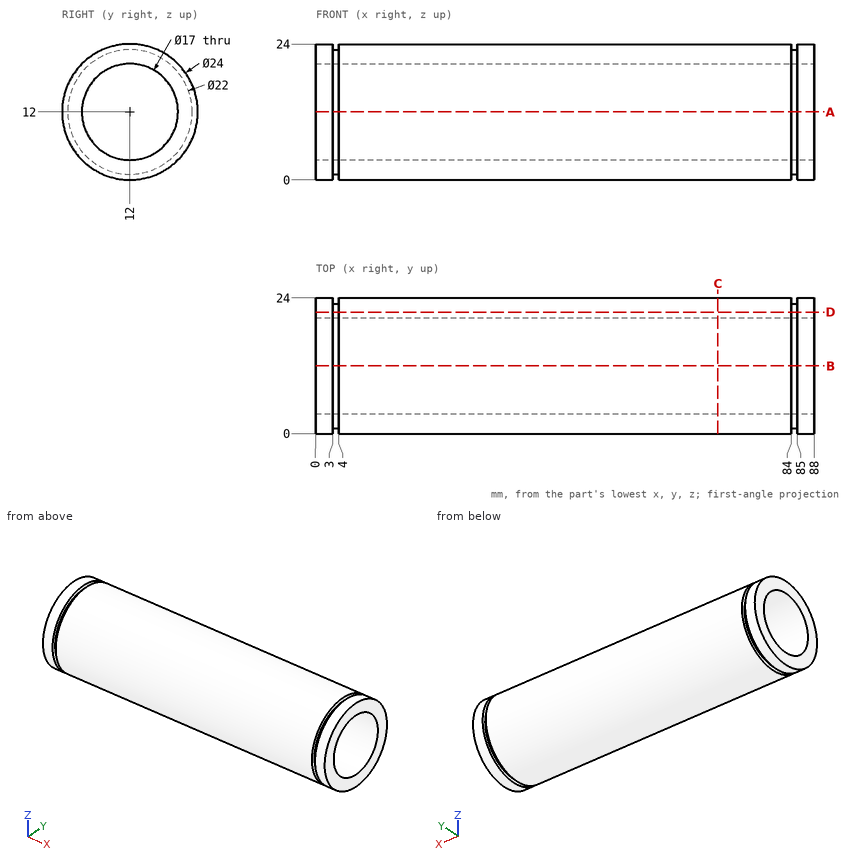
Design review of the part shown in the three views and the two pictorial views. Dimensions are in mm from the part's minimum x, y and z. Coordinates: 2 decimals unless noted, no trailing zeros. Order: outer loops, then holes, each group sorted by start corner. A loop starts at its lowest first (then second) coordinate and runs counter-clockwise, first axis right, second up.
1) Take a section at C-C, the plane x = 71. Give the boundary of the cut face in (y, z).
2) Take a section at A-A, the plane z = 12. Give the boundary of the cut face in (x, y).
3) Wall thickness on line 1 along X through (y, z) = (20.25, 20.5); line 2 along Y through (x, z) = (39.5, 11.5); line 3 along Z through (x, y) = (46.5, 9.5): over which ranges is each line inside the solid? List them lowest first.
4) Clearance check with flat-ended pins moving along their axes: pin 1 (10 mm diameter, centred on y = 12, z = 12, fed in from +X); pin 2 (10 mm diameter, centred on x = 41.5, y = 3, fed in from +Z); pin 3 (6 mm diameter, centred on x = 64.5, y = 20, fed in from +Z); pin 4 (8 mm diameter, centred on x = 61.5, y = 18, fed in from -Z). State where each tip first meets the part, or that it passes through.
5) Take a section at D-D, the plane y = 21.5. Give the boundary of the cut face in (x, z).
Returned:
1. outline: circle Ø24 at (12, 12); hole circle Ø17 at (12, 12)
2. outline: (0, 0) - (3, 0) - (3, 1) - (4, 1) - (4, 0) - (84, 0) - (84, 1) - (85, 1) - (85, 0) - (88, 0) - (88, 3.5) - (0, 3.5) - close; (0, 20.5) - (88, 20.5) - (88, 24) - (85, 24) - (85, 23) - (84, 23) - (84, 24) - (4, 24) - (4, 23) - (3, 23) - (3, 24) - (0, 24) - close
3. line 1: x = 0 to 3, 4 to 84, 85 to 88
3. line 2: y = 0.01 to 3.51, 20.49 to 23.99
3. line 3: z = 0.26 to 3.88, 20.12 to 23.74
4. pin 1: passes through
4. pin 2: stops at z = 23.31
4. pin 3: stops at z = 22.91
4. pin 4: stops at z = 0.17
5. outline: (0, 4.67) - (3, 4.67) - (3, 6.45) - (4, 6.45) - (4, 4.67) - (84, 4.67) - (84, 6.45) - (85, 6.45) - (85, 4.67) - (88, 4.67) - (88, 19.33) - (85, 19.33) - (85, 17.55) - (84, 17.55) - (84, 19.33) - (4, 19.33) - (4, 17.55) - (3, 17.55) - (3, 19.33) - (0, 19.33) - close
